```python
from build123d import *

# Parameters (mm, degrees)
F0_W     = 50.8
F0_H     = 101.6
F1_DEPTH = 101.6
F2_T     = -6.35
F4_D     = 12.7
F6_D     = 25.4
F6_DEPTH = 25.4
F8_D     = 8.001


with BuildPart() as f1:
    # F0 (on Top) → F1 (new body)
    with BuildSketch(Plane.XY):
        Rectangle(F0_W, F0_H)
    extrude(amount=F1_DEPTH)

    # F2
    f2_openings = [f1.faces().sort_by_distance(p)[0] for p in [
        (0, 0, 101.6),
    ]]
    offset(amount=F2_T, openings=f2_openings)

    # F4 (through all)
    with Locations(Plane.YZ.offset(25.4)):
        with Locations((0, 76.2)):
            Hole(F4_D / 2)

    # F6
    with Locations(Plane(origin=(0, 0, 0), x_dir=(1, 0, 0), z_dir=(0, 0, -1))):
        with Locations((0, 0)):
            Hole(F6_D / 2, depth=F6_DEPTH)

    # F8 (through all)
    with Locations(Plane.XZ.offset(50.8)):
        with Locations((0, 50.8)):
            Hole(F8_D / 2)


solid = f1.part
```
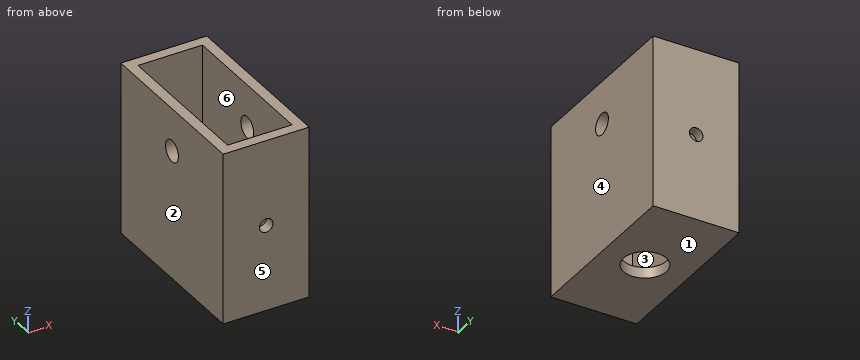
For this review, take the finished solid that the model builds, in its own axes (mm). Face numbers are marked on the shaded views. A direction names the side the tool comes from. Round coordinates to 2 decimals unless told otherwise and drop trailing zeros. Order: outer loops, then holes, each group sorted by start corner. A loop starts at its lowest first (then second) coordinate and runs counter-clockwise, first axis right, second up.
Q1. We need section A-A, the plane z = 50.8. Give the boundary of the cut face in (x, y), plus the area to 3 significant figures.
Findings below:
outline: (-25.4, -50.8) - (-4, -50.8) - (-4, -44.45) - (-19.05, -44.45) - (-19.05, 44.45) - (-4, 44.45) - (-4, 50.8) - (-25.4, 50.8) - close; (4, -50.8) - (25.4, -50.8) - (25.4, 50.8) - (4, 50.8) - (4, 44.45) - (19.05, 44.45) - (19.05, -44.45) - (4, -44.45) - close
area: 1,670 mm2
Q2. We need section B-B, the plane x = 10. Give the boundary of the cut face in (y, z).
Findings below:
outline: (-50.8, 0) - (-7.83, 0) - (-7.83, 6.35) - (-44.45, 6.35) - (-44.45, 101.6) - (-50.8, 101.6) - close; (7.83, 0) - (50.8, 0) - (50.8, 101.6) - (44.45, 101.6) - (44.45, 6.35) - (7.83, 6.35) - close
Q3. Machinability: for the marked faces 5 and 6, which of the approach directions +Z, -Z, +X, -X, +Y, -Y give a long, thin tool a straight path to every point of the face, cutting with its end or side? Answer none if there is none.
Findings below:
face 5: +Z, -Z, +X, -X, -Y
face 6: +Z
Q4. We need section D-D, the plane y = -43. Give the boundary of the cut face in (x, z).
Findings below:
outline: (-25.4, 0) - (25.4, 0) - (25.4, 101.6) - (19.05, 101.6) - (19.05, 6.35) - (-19.05, 6.35) - (-19.05, 101.6) - (-25.4, 101.6) - close
Q5. Insertion check: P1, Ø12, axis at x = -17, y = -40, coming from the +Z side; P2, Ø12, axis at x = -0.5, y = 8.5, coming from the +Z side. Each pin has a flat end and moves straight along its axis. Give the tip position at first contact, or say it passes through.
Findings below:
P1: stops at z = 101.6
P2: stops at z = 6.35
Q6. Wall thickness on line 1 (Y direction, x = -9.5, z = 33); line 2 (X direction, y = 32, z = 97); line 3 (Z direction, x = 0, y = 48): over which ranges is each line inside the solid? List them lowest first.
Findings below:
line 1: y = -50.8 to -44.45, 44.45 to 50.8
line 2: x = -25.4 to -19.05, 19.05 to 25.4
line 3: z = 0 to 46.8, 54.8 to 101.6
Q7. Mouldability with a two-part tool opening along X and no side actions: class the marked faces 1, 2, 3 and 4 as pulls with the +X half, pulls with the -X half, needs draft (parallel to the pull), parting line crosses it, or undercut.
Findings below:
face 1: needs draft
face 2: pulls with the -X half
face 3: undercut
face 4: pulls with the +X half
Q8. We need section C-C, the plane y = -2. Give the boundary of the cut face in (x, z), plus the area to 3 significant figures.
Findings below:
outline: (-25.4, 0) - (-12.54, 0) - (-12.54, 6.35) - (-19.05, 6.35) - (-19.05, 70.17) - (-25.4, 70.17) - close; (-25.4, 82.23) - (-19.05, 82.23) - (-19.05, 101.6) - (-25.4, 101.6) - close; (12.54, 0) - (25.4, 0) - (25.4, 70.17) - (19.05, 70.17) - (19.05, 6.35) - (12.54, 6.35) - close; (19.05, 82.23) - (25.4, 82.23) - (25.4, 101.6) - (19.05, 101.6) - close
area: 1,220 mm2
